Work out the finished part from the listing and answer in its coordinate system (mm). Round coordinates to 2 decimals unless told otherwise and drop trailing zeros. Order: outer loops, then holes, each group sorted by start corner. A loop starts at its lowest first (then second) coordinate and runs counter-clockwise, first axis right, second up. Notation, with made-up numbers: (82.25, -18.75) -> (128.25, -18.75) arc R6 ccw to (128.25, -10.75) -> close; hole circle Ø4 at (30.5, -17.5). An arc over 180 degrees is marked (long way). Use one line per item in the form item = value.
```python
from build123d import *

# Parameters (mm, degrees)
F0_W      = 254
F0_H      = 152.4
F1_DEPTH  = 12.7
F2_W      = 50.8
F2_H      = 50.8
F3_DEPTH  = 6.35
F4_W      = 50.8
F4_H      = 6.35
F5_DEPTH  = 44.45
F7_DEPTH  = 25.4
F9_DEPTH  = 12.7
F10_W     = 76.2
F10_H     = 12.7
F11_DEPTH = 38.1
F13_DEPTH = 50.8
F14_W     = 38.1
F14_H     = 38.1
F15_DEPTH = 647.7
F16_W     = 25.4
F16_H     = 25.4
F17_DEPTH = 203.2
F18_W     = 25.4
F18_H     = 76.2
F19_DEPTH = 12.7
F20_W     = 25.4
F20_H     = 76.2
F21_DEPTH = 12.7


with BuildPart() as f1:
    # F0 (on Top) → F1 (new body)
    with BuildSketch(Plane.XY):
        with Locations((130.337225, 76.2)):
            Rectangle(F0_W, F0_H)
    extrude(amount=F1_DEPTH)

    # F2 (on face) → F3 (join)
    with BuildSketch(Plane.XY.offset(12.7)):
        with Locations((130.337225, 114.3)):
            Rectangle(F2_W, F2_H)
    extrude(amount=F3_DEPTH)

    # F4 (on face) → F5 (join)
    with BuildSketch(Plane.XY.offset(19.05)):
        with Locations((130.337225, 92.075)):
            Rectangle(F4_W, F4_H)
    extrude(amount=F5_DEPTH)

    # F6 (on face) → F7 (cut)
    with BuildSketch(Plane.XY.offset(12.7)):
        with BuildLine():
            ThreePointArc((158.735288, 76.2), (157.975611, 82.724538), (155.737225, 88.9))
            Line((155.737225, 88.9), (104.937225, 88.9))
            ThreePointArc((104.937225, 88.9), (123.812687, 48.561614), (158.735288, 76.2))
        make_face()
        with BuildLine():
            Line((104.937225, 88.9), (155.737225, 88.9))
            ThreePointArc((155.737225, 88.9), (130.337225, 104.598063), (104.937225, 88.9))
        make_face()
    extrude(amount=-F7_DEPTH, mode=Mode.SUBTRACT)

    # F8 (on face) → F9 (join)
    with BuildSketch(Plane(origin=(0, 0, 0), x_dir=(1, 0, 0), z_dir=(0, 0, -1))):
        Polygon((92.237225, -152.4), (130.337225, -152.4), (168.437225, -152.4), (168.437225, -101.6), (92.237225, -101.6), align=None)
    extrude(amount=F9_DEPTH)

    # F10 (on face) → F11 (join)
    with BuildSketch(Plane(origin=(0, 0, -12.7), x_dir=(1, 0, 0), z_dir=(0, 0, -1))):
        with Locations((130.337225, -146.05)):
            Rectangle(F10_W, F10_H)
    extrude(amount=F11_DEPTH)

    # F12 (on face) → F13 (join)
    with BuildSketch(Plane(origin=(0, 152.4, 0), x_dir=(-1, 0, 0), z_dir=(0, 1, 0))):
        Polygon((-104.937225, 203.2), (-130.337225, 203.2), (-155.737225, 203.2), (-155.737225, -406.4), (-104.937225, -406.4), align=None)
    extrude(amount=F13_DEPTH)

    # F14 (on face) → F15 (cut)
    with BuildSketch(Plane(origin=(0, 0, -406.4), x_dir=(1, 0, 0), z_dir=(0, 0, -1))):
        with Locations((130.337225, -177.8)):
            Rectangle(F14_W, F14_H)
    extrude(amount=-F15_DEPTH, mode=Mode.SUBTRACT)

    # F16 (on face) → F17 (join)
    with BuildSketch(Plane.XY.offset(12.7)):
        with Locations((16.037225, 114.3)):
            Rectangle(F16_W, F16_H)
        with Locations((244.637225, 114.3)):
            Rectangle(F16_W, F16_H)
    extrude(amount=F17_DEPTH)

    # F18 (on face) → F19 (join)
    with BuildSketch(Plane.XY.offset(215.9)):
        with Locations((244.637225, 88.9)):
            Rectangle(F18_W, F18_H)
    extrude(amount=F19_DEPTH)

    # F20 (on face) → F21 (join)
    with BuildSketch(Plane.XY.offset(215.9)):
        with Locations((16.037225, 88.9)):
            Rectangle(F20_W, F20_H)
    extrude(amount=F21_DEPTH)


solid = f1.part
```
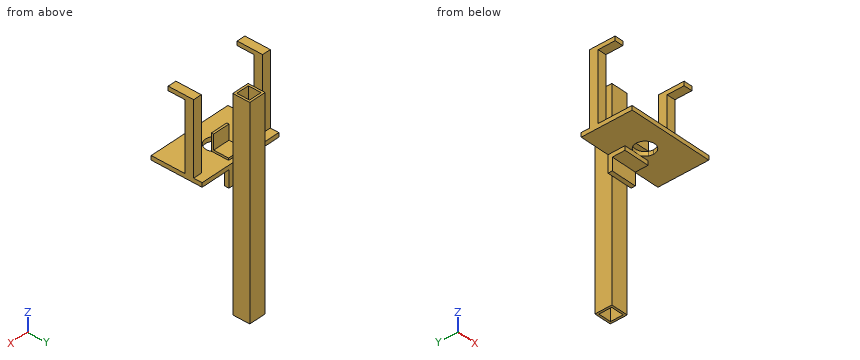
Item 1: Consider line 1 along X through (y, z) = (76.2, 7.25); line 2 along Y through (x, z) = (131, -195.5); line 3 along Z through (x, y) = (227, 140). Determine where each line is inside the solid, lowest interval first.
Findings:
line_1 = 3.34 to 101.94, 158.74 to 257.34
line_2 = 152.4 to 158.75, 196.85 to 203.2
line_3 = 0 to 12.7
Item 2: The part is cut by section B-B, the plane y = 188.5. Give the vertices of the cut face in (x, z).
Findings:
outline = (104.94, -406.4) -> (111.29, -406.4) -> (111.29, 203.2) -> (104.94, 203.2) -> close; (149.39, -406.4) -> (155.74, -406.4) -> (155.74, 203.2) -> (149.39, 203.2) -> close
Item 3: Flat-ended cylindrical pins translate along their axes: P1, Ø15, axis at y = 172.5, z = -143, coming from the +X side; P2, Ø12, axis at x = 30.5, y = 70.5, coming from the +Z side; P3, Ø1.5, axis at x = 146, y = 94, coming from the +Z side; P4, Ø7.5, axis at x = 18, z = 92.5, coming from the +Y side. Find the tip coordinate at first contact, or state that the pin passes through.
Findings:
P1 = 155.74
P2 = 228.6
P3 = 63.5
P4 = 127
Item 4: The part is cut by section A-A, the plane z = -248.5. Give the vertices of the cut face in (x, y), and give its area (3 significant figures).
Findings:
outline = (104.94, 152.4) -> (155.74, 152.4) -> (155.74, 203.2) -> (104.94, 203.2) -> close; hole (111.29, 158.75) -> (149.39, 158.75) -> (149.39, 196.85) -> (111.29, 196.85) -> close
area = 1,130 mm^2
Item 5: The part is cut by section D-D, the plane y = 30. Give the vertices of the cut face in (x, z), and give its area (3 significant figures).
Findings:
outline = (3.34, 0) -> (257.34, 0) -> (257.34, 12.7) -> (3.34, 12.7) -> close
area = 3,230 mm^2
Item 6: The part is cut by section C-C, the plane x = 239.5. Give the vertices of the cut face in (y, z), and give its area (3 significant figures).
Findings:
outline = (0, 0) -> (152.4, 0) -> (152.4, 12.7) -> (127, 12.7) -> (127, 228.6) -> (50.8, 228.6) -> (50.8, 215.9) -> (101.6, 215.9) -> (101.6, 12.7) -> (0, 12.7) -> close
area = 8,060 mm^2
